from build123d import *

# Parameters (mm, degrees)
EXTRUDE_1_DEPTH     = 40
SKETCH_3_R          = 0.5
CUT_EXTRUDE_1_DEPTH = 40
EXTRUDE_START       = -40
EXTRUDE_5_DEPTH     = 40
EXTRUDE_6_DEPTH     = 40
SKETCH_14_W         = 2.5
SKETCH_14_H         = 8
CUT_EXTRUDE_8_DEPTH = 40
SKETCH_15_W         = 3
SKETCH_15_H         = 4
CUT_EXTRUDE_9_DEPTH = 41.71781145
SKETCH_16_W         = 0.8
SKETCH_16_H         = 0.8
EXTRUDE_7_DEPTH     = 40
SKETCH_17_W         = 3
SKETCH_17_H         = 2
EXTRUDE_8_DEPTH     = 1
SKETCH_18_W         = 3
SKETCH_18_H         = 2
EXTRUDE_9_DEPTH     = 1


with BuildPart() as part:
    # 草图2 → 凸台-拉伸1 (new body)
    with BuildSketch(Plane.XY):
        with BuildLine():
            Line((-1.655607757, 0), (6.344392243, 0))
            ThreePointArc((6.344392243, 0), (7.344397132, 0.999995111), (6.344402021, 2))
            Line((6.344402021, 2), (-1.655607757, 2))
            ThreePointArc((-1.655607757, 2), (-2.655607757, 1), (-1.655607757, 0))
        make_face()
    extrude(amount=EXTRUDE_1_DEPTH)

    # 草图3 → 切除-拉伸1 (cut)
    with BuildSketch(Plane.XY.offset(40)):
        with Locations((-1.655607757, 1)):
            Circle(SKETCH_3_R)
        with Locations((6.344392243, 1.020580345)):
            Circle(SKETCH_3_R)
    extrude(amount=-CUT_EXTRUDE_1_DEPTH, mode=Mode.SUBTRACT)

    # 草图11 → 凸台-拉伸5 (add)
    with BuildSketch(Plane.XY.offset(40).offset(EXTRUDE_START)):
        with BuildLine():
            Line((-1.655607757, 2.8), (-0.655607757, 2.8))
            Line((-0.655607757, 2.8), (-0.655607757, 2))
            Line((-0.655607757, 2), (-1.655607757, 2))
            ThreePointArc((-1.655607757, 2), (-2.127012277, 1.881917104), (-2.487087176, 1.555555556))
            Line((-2.487087176, 1.555555556), (-1.655607757, 2.8))
        make_face()
    extrude(amount=EXTRUDE_5_DEPTH)

    # 草图12 → 凸台-拉伸6 (add)
    with BuildSketch(Plane.XY.offset(40).offset(EXTRUDE_START)):
        with BuildLine():
            Line((6.231808662, 1.993641704), (5.701534493, 2))
            Line((5.701534493, 2), (6.231808662, 2.793641704))
            Line((6.231808662, 2.793641704), (7.231808662, 2.793641704))
            Line((7.231808662, 2.793641704), (7.231808662, 1.993641704))
            Line((7.231808662, 1.993641704), (7.335350835, 1.134204168))
            ThreePointArc((7.335350835, 1.134204168), (7.043760809, 1.71476601), (6.456985603, 1.993641704))
            Line((6.456985603, 1.993641704), (6.231808662, 1.993641704))
        make_face()
    extrude(amount=EXTRUDE_6_DEPTH)

    # 草图14 → 切除-拉伸8 (cut)
    with BuildSketch(Plane(origin=(0, 0, 0), x_dir=(1, 0, 0), z_dir=(0, 1, 0))):
        with Locations((-1.405607757, -12)):
            Rectangle(SKETCH_14_W, SKETCH_14_H)
        with Locations((-1.405607757, -28)):
            Rectangle(SKETCH_14_W, SKETCH_14_H)
        with Locations((6.094397132, -4)):
            Rectangle(SKETCH_14_W, SKETCH_14_H)
        with Locations((6.094397132, -20)):
            Rectangle(SKETCH_14_W, SKETCH_14_H)
        with Locations((6.094397132, -36)):
            Rectangle(SKETCH_14_W, SKETCH_14_H)
    extrude(amount=CUT_EXTRUDE_8_DEPTH, mode=Mode.SUBTRACT)

    # 草图15 → 切除-拉伸9 (cut, through all)
    with BuildSketch(Plane(origin=(0, 2, 0), x_dir=(1, 0, 0), z_dir=(0, 1, 0))):
        with Locations((2.344392243, -14)):
            Rectangle(SKETCH_15_W, SKETCH_15_H)
        with Locations((2.344392243, -26)):
            Rectangle(SKETCH_15_W, SKETCH_15_H)
    extrude(amount=-CUT_EXTRUDE_9_DEPTH, mode=Mode.SUBTRACT)

    # 草图16 → 凸台-拉伸7 (add)
    with BuildSketch(Plane.XY.offset(40)):
        with Locations((4.444397132, 2.4)):
            Rectangle(SKETCH_16_W, SKETCH_16_H)
    extrude(amount=-EXTRUDE_7_DEPTH)

    # 草图17 → 凸台-拉伸8 (add)
    with BuildSketch(Plane.XY.offset(24)):
        with Locations((2.344392243, -1)):
            Rectangle(SKETCH_17_W, SKETCH_17_H)
    extrude(amount=-EXTRUDE_8_DEPTH)

    # 草图18 → 凸台-拉伸9 (add)
    with BuildSketch(Plane(origin=(0, 0, 16), x_dir=(-1, 0, 0), z_dir=(0, 0, -1))):
        with Locations((-2.344392243, -1)):
            Rectangle(SKETCH_18_W, SKETCH_18_H)
    extrude(amount=-EXTRUDE_9_DEPTH)


solid = part.part
Verification items for the finished model (mm, model axes). A direction names the side the tool comes from. Coordinates: 2 decimals unless noted, no trailing zeros. Order: outer loops, then holes, each group sorted by start corner. A loop starts at its lowest first (then second) coordinate and runs counter-clockwise, first axis right, second up.
Item 1: Section check B-B, the plane y = -0.8. Enter the section's corners in (x, z), then the cut area to 3 significant figures.
Filled in:
outline: (0.84, 16) - (3.84, 16) - (3.84, 17) - (0.84, 17) - close; (0.84, 23) - (3.84, 23) - (3.84, 24) - (0.84, 24) - close
area: 6.00 mm2
Item 2: Depth check by flat-ended pin: pin 1 (1 mm diameter, centred on x = 6, y = 2, fed in from -Z); pin 2 (1.5 mm diameter, centred on x = 0.5, z = 33.5, fed in from -Y); pin 3 (1 mm diameter, centred on y = 0.5, z = 12.5, fed in from -X). Enter the tip coordinate at first touch or a pass-through.
Filled in:
pin 1: stops at z = 8
pin 2: stops at y = 0
pin 3: stops at x = -0.16
Item 3: Access from +Z, -Z, +X, -X, +Y, -Y to the whole of each face (thin tool, end or side, straight path). Record for faces 1 (the face through (5.8, 1.4, 16)), 2 (the face through (4.844, 2, 20)), 3 (the face through (5, 2, 12)), 4 (the face through (3.844, -1, 23.5)).
Filled in:
face 1: +X, +Y, -Y
face 2: +Y
face 3: +Z, -Z, +Y
face 4: +Z, -Z, +X, -Y
Item 4: Section check D-D, the plane z = 15.5. Enter the section's corners in (x, y), then the cut area to 3 significant figures.
Filled in:
outline: (-0.16, 0) - (0.84, 0) - (0.84, 2) - (-0.16, 2) - close; (3.84, 0) - (6.34, 0) arc R1 ccw to (7.34, 1.13) - (7.23, 1.99) - (7.23, 2.79) - (6.23, 2.79) - (5.7, 2) - (4.84, 2) - (4.84, 2.8) - (4.04, 2.8) - (4.04, 2) - (3.84, 2) - close; hole circle Ø1 at (6.34, 1.02)
area: 9.59 mm2
Item 5: Material ranges on L1, parallel to Z at x = 2, y = 0.3; L2, parallel to X at y = 0.95, z = 27.5; L3, parallel to Z at x = -2, y = 1.6, recorded low to high.
Filled in:
L1: z = 0 to 12, 16 to 24, 28 to 40
L2: x = -0.16 to 0.84, 3.84 to 5.85, 6.84 to 7.34
L3: z = 0 to 8, 16 to 24, 32 to 40
Item 6: Section check C-C, the plane z = 7. Enter the section's corners in (x, y), then the cut area to 3 significant figures.
Filled in:
outline: (-2.49, 1.56) arc R1 ccw to (-1.66, 0) - (4.84, 0) - (4.84, 2.8) - (4.04, 2.8) - (4.04, 2) - (-0.66, 2) - (-0.66, 2.8) - (-1.66, 2.8) - close; hole circle Ø1 at (-1.66, 1)
area: 15.5 mm2
Item 7: Release check for a two-part mould opening along Z. For faces 5 (the face through (-2.077, 2.169, 3.944)), 6 (the face through (-0.156, 1, 28)), 7 (the face through (1, 1, 0)) record: +Z half, -Z half, draft (parallel to the pull), parting line (faces both ways), or undercut.
Filled in:
face 5: draft
face 6: undercut
face 7: -Z half
Item 8: Section check A-A, the plane x = 2.5. Enter the section's corners in (y, z).
Filled in:
outline: (-2, 16) - (2, 16) - (2, 24) - (-2, 24) - (-2, 23) - (0, 23) - (0, 17) - (-2, 17) - close; (0, 0) - (2, 0) - (2, 12) - (0, 12) - close; (0, 28) - (2, 28) - (2, 40) - (0, 40) - close
